```python
from build123d import *

# Parameters (mm, degrees)
SKETCH1_W           = 42
SKETCH1_H           = 18
BOSS_EXTRUDE1_DEPTH = 8
FILLET1_R           = 5
FILLET2_R           = 2
SHELL1_START        = -7
SHELL1_DEPTH        = 14
SKETCH2_R           = 7
CUT_EXTRUDE1_DEPTH  = 25.207436874


# Read off the part's stored shape, not the designer's step: Shell1
with BuildPart() as part:
    # Sketch1 → Boss-Extrude1 (new body)
    with BuildSketch(Plane.XY):
        Rectangle(SKETCH1_W, SKETCH1_H)
    extrude(amount=BOSS_EXTRUDE1_DEPTH)

    # Fillet1
    fillet1_edges = [part.edges().sort_by_distance(p)[0] for p in [
        (21, 0, 8),
        (-21, 0, 8),
    ]]
    fillet(fillet1_edges, radius=FILLET1_R)

    # Fillet2
    fillet2_edges = [part.edges().sort_by_distance(p)[0] for p in [
        (0, -9, 8),
        (0, 9, 8),
        (21, -9, 1.5),
        (-21, -9, 1.5),
        (19.535533906, -9, 6.535533906),
        (-19.535533906, -9, 6.535533906),
        (-21, 9, 1.5),
        (21, 9, 1.5),
        (19.535533906, 9, 6.535533906),
        (-19.535533906, 9, 6.535533906),
    ]]
    fillet(fillet2_edges, radius=FILLET2_R)

    # Shell1 outline → Shell1 (cut)
    with BuildSketch(Plane(origin=(0, 0, 0), x_dir=(1, 0, 0), z_dir=(0, 1, 0)).offset(SHELL1_START)):
        with BuildLine():
            Line((-19, 0), (-19, -3))
            ThreePointArc((-19, -3), (-18.121320344, -5.121320344), (-16, -6))
            Line((-16, -6), (16, -6))
            ThreePointArc((16, -6), (18.121320344, -5.121320344), (19, -3))
            Line((19, -3), (19, 0))
            Line((19, 0), (-19, 0))
        make_face()
    extrude(amount=SHELL1_DEPTH, mode=Mode.SUBTRACT)

    # Sketch2 → Cut-Extrude1 (cut, through all)
    with BuildSketch(Plane.XY.offset(8)):
        with Locations(Location((0, 0, 0), (0, 0, 270))):
            Circle(SKETCH2_R)
    extrude(amount=-CUT_EXTRUDE1_DEPTH, mode=Mode.SUBTRACT)


solid = part.part
```
Could you check a few things on this model? Use its own coordinates, in mm. A direction names the side the tool comes from. Round coordinates to 2 decimals unless told otherwise and drop trailing zeros. Loops run counter-clockwise (first coordinate to the right, second up) from the corner with the lowest first, then second, coordinate; pieces in that order, holes last. Notation, with made-up numbers: (56.25, 29) - (78.25, 29) arc R18 cw to (78.25, 49) - close; hole circle Ø1 at (15.25, 38). An arc over 180 degrees is marked (long way). Answer in a Markdown table with one row per item. Add a question column.
(1) I need wall thicknesses on line 1 along X through (y, z) = (1, 0.5); line 2 along Y through (x, z) = (1.5, 2.5); line 3 along Z through (x, y) = (10.5, -2.75). Which ranges of each line are inside material? Lowest first, please.
(2) If we section it at A-A (z = 1.25): Please give me the cut outline in (x, y).
(3) If we mould it in two halves opening along Y, with no side actions, what happens to faces 1 (the face through (-18.14, -0.1, 5.1)), 2 (the face through (0.22, 8.43, 7.4)), 3 (the face through (21, 0, 1))? For each: pulls with the +Y half, pulls with the -Y half, needs draft (parallel to the pull), parting line crosses it, or undercut.
(4) If we section it at B-B (x = 2.5): Please give me the cut outline in (y, z).
(5) I'm going to push a flat-ended pin straight in: pin 1 (4 mm diameter, centred on x = 10.5, y = -2.5, fed in from -Z). Where does the tip first touch, or does it pass through?
(6) For faces 4 (the face through (-20.4, 8.43, 1.52)), 5 (the face through (19, 0, 2)), which set-ups out of +Z, -Z, +X, -X, +Y, -Y let a thin tool reach every point of the face, with its end or its side?
(7) If we section it at D-D (x = -13.5): Please give me the cut outline in (y, z).
(8) If we section it at C-C (y = 0): Please give me the cut outline in (x, z).
Model answer:
| question | item | result |
|---|---|---|
| 1 | line 1 | x = -21 to -19, 19 to 21 |
| 1 | line 2 | y = -9 to -7, 7 to 9 |
| 1 | line 3 | z = 6 to 8 |
| 2 | outline | (-21, -7) arc R2 ccw to (-19, -9) - (19, -9) arc R2 ccw to (21, -7) - (21, 7) arc R2 ccw to (19, 9) - (-19, 9) arc R2 ccw to (-21, 7) - close; hole (-19, -7) - (19, -7) - (19, 7) - (-19, 7) - close |
| 3 | face 1 | undercut |
| 3 | face 2 | pulls with the +Y half |
| 3 | face 3 | needs draft |
| 4 | outline | (-9, 0) - (-7, 0) - (-7, 6) - (-6.54, 6) - (-6.54, 8) - (-7, 8) arc R2 ccw to (-9, 6) - close; (6.54, 6) - (7, 6) - (7, 0) - (9, 0) - (9, 6) arc R2 ccw to (7, 8) - (6.54, 8) - close |
| 5 | pin 1 | stops at z = 6 |
| 6 | face 4 | +Z, -Z, -X, +Y |
| 6 | face 5 | -Z |
| 7 | outline | (-9, 0) - (-7, 0) - (-7, 6) - (7, 6) - (7, 0) - (9, 0) - (9, 6) arc R2 ccw to (7, 8) - (-7, 8) arc R2 ccw to (-9, 6) - close |
| 8 | outline | (-21, 0) - (-19, 0) - (-19, 3) arc R3 cw to (-16, 6) - (-7, 6) - (-7, 8) - (-16, 8) arc R5 ccw to (-21, 3) - close; (7, 6) - (16, 6) arc R3 cw to (19, 3) - (19, 0) - (21, 0) - (21, 3) arc R5 ccw to (16, 8) - (7, 8) - close |
